Geometry check sheet. Reference: drawing and pictorial views, mm from the part's lowest x, y, z. A direction names the side the tool comes from. Round coordinates to 2 decimals unless told otherwise and drop trailing zeros. Order: outer loops, then holes, each group sorted by start corner. A loop starts at its lowest first (then second) coordinate and runs counter-clockwise, first axis right, second up. Notation, with made-up numbers: (2.5, -10.5) -> (29.5, -10.5) arc R19 ccw to (29.5, -4.5) -> close; hole circle Ø4 at (-16, 1.25). An arc over 180 degrees is marked (long way). Return JSON: item names as keys, results as strings. Group by question number.
1) Section check A-A on z = 14.5. Enter the section's corners in (x, y).
2) Scan lines: L1, parallel to Y at x = 46.5, z = 21.5; L2, parallel to X at y = 37, z = 15.5; L3, parallel to Z at x = 64.5, y = 10. Record each from-to range of solid material in increasing order.
3) Tool access check on the marked faces 1 and 2. Record the directions out of +Z, -Z, +X, -X, +Y, -Y that give a thin tool (end or side, any length) a straight path to the whole face; none if there is none.
4) Section check C-C on y = 38. Enter the section's corners in (x, z).
5) Section check B-B on x = 47.5. Enter the section's corners in (y, z), plus the area to 3 significant figures.
6) Depth check by flat-ended pin: pin 1 (4.5 mm diameter, centred on y = 23.5, z = 1, fed in from +X); pin 2 (3 mm diameter, centred on x = 37.5, z = 1.5, fed in from +Y). Enter the tip coordinate at first touch or a pass-through.
7) Draft check along Y on the marked faces 3, 4, 5 and 6. Enter one of: pulls with the +Y half, pulls with the -Y half, needs draft (parallel to the pull), parting line crosses it, or undercut.
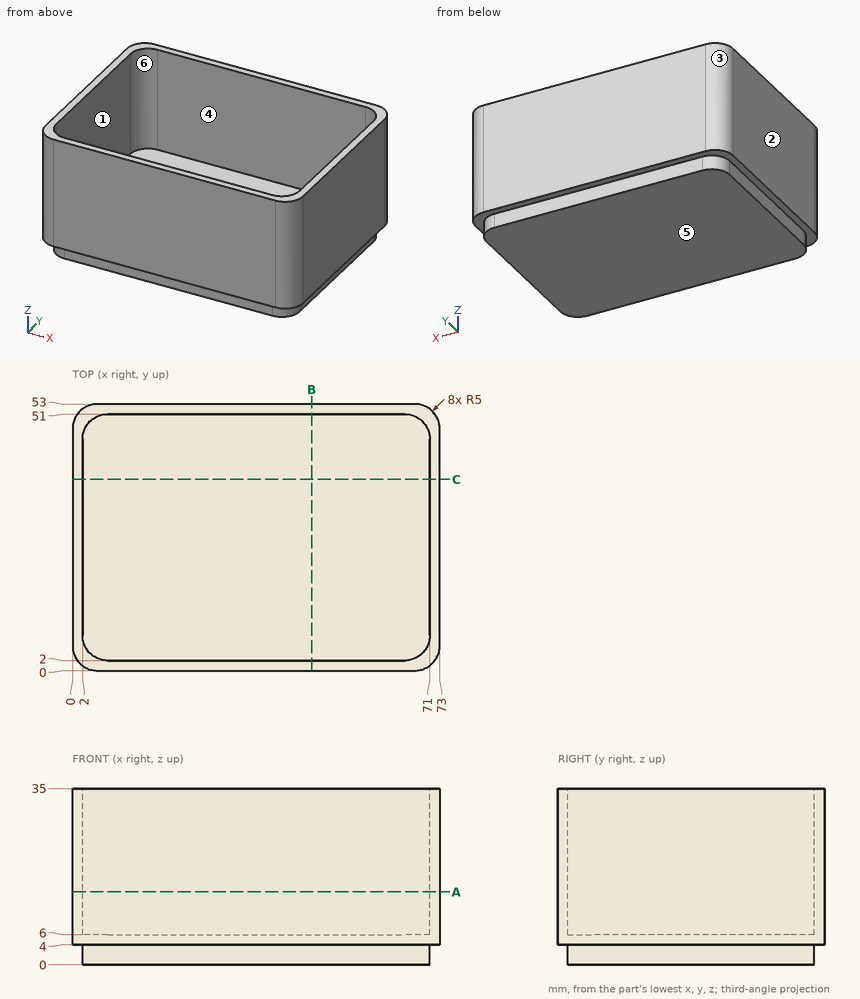
Check result:
{
 "1": {"outline": "(0, 5) arc R5 ccw to (5, 0) -> (68, 0) arc R5 ccw to (73, 5) -> (73, 48) arc R5 ccw to (68, 53) -> (5, 53) arc R5 ccw to (0, 48) -> close; hole (2, 7) arc R5 ccw to (7, 2) -> (66, 2) arc R5 ccw to (71, 7) -> (71, 46) arc R5 ccw to (66, 51) -> (7, 51) arc R5 ccw to (2, 46) -> close"},
 "2": {"L1": "0 to 2, 51 to 53", "L2": "0 to 2, 71 to 73", "L3": "0 to 6"},
 "3": {"face 1": "+Z", "face 2": "+Z, -Z, -X, +Y, -Y"},
 "4": {"outline": "(0, 4) -> (2, 4) -> (2, 0) -> (71, 0) -> (71, 4) -> (73, 4) -> (73, 35) -> (71, 35) -> (71, 6) -> (2, 6) -> (2, 35) -> (0, 35) -> close"},
 "5": {"outline": "(0, 4) -> (2, 4) -> (2, 0) -> (51, 0) -> (51, 4) -> (53, 4) -> (53, 35) -> (51, 35) -> (51, 6) -> (2, 6) -> (2, 35) -> (0, 35) -> close", "area": "418 mm^2"},
 "6": {"pin 1": "x = 71", "pin 2": "y = 51"},
 "7": {"face 3": "pulls with the +Y half", "face 4": "undercut", "face 5": "needs draft", "face 6": "undercut"}
}
